Read the model definition and answer for the solid it produces. Units are mm, in the model's axes. Face numbers are marked on the shaded views. A direction names the side the tool comes from. Coordinates: 2 decimals unless noted, no trailing zeros. Loops run counter-clockwise (first coordinate to the right, second up) from the corner with the lowest first, then second, coordinate; pieces in that order, holes last. Notation, with made-up numbers: M 66.5,-20.75 L 71.5,-20.75 A27 ccw 71.5,5.25 Z; hole C -32,29.25 d4. An arc over 180 degrees is marked long. Put each result on its own line as item: value.
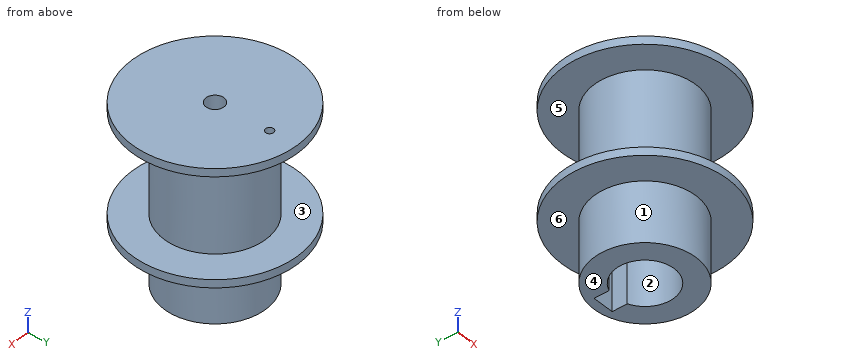
from build123d import *

# Parameters (mm, degrees)
SKETCH1_R           = 12.7
BOSS_EXTRUDE1_DEPTH = 28
SKETCH3_R           = 20.7
SKETCH3_R_2         = 12.7
BOSS_EXTRUDE2_DEPTH = 2
SKETCH4_R           = 12.7
SKETCH4_R_2         = 2.25
BOSS_EXTRUDE3_DEPTH = 14
SKETCH5_R           = 20.7
SKETCH5_R_2         = 2.25
SKETCH5_R_3         = 1
BOSS_EXTRUDE4_DEPTH = 2


with BuildPart() as part:
    # Sketch1 → Boss-Extrude1 (new body)
    with BuildSketch(Plane.XY):
        Circle(SKETCH1_R)
        with BuildLine():
            Line((-2.7, 6.728484228), (-2.7, 10.5))
            Line((-2.7, 10.5), (2.7, 10.5))
            Line((2.7, 10.5), (2.7, 6.728484228))
            ThreePointArc((2.7, 6.728484228), (0, -7.25), (-2.7, 6.728484228))
        make_face(mode=Mode.SUBTRACT)
    extrude(amount=BOSS_EXTRUDE1_DEPTH)

    # Sketch3 → Boss-Extrude2 (add)
    with BuildSketch(Plane(origin=(0, 0, 15), x_dir=(-1, 0, 0), z_dir=(0, 0, -1))):
        Circle(SKETCH3_R)
        Circle(SKETCH3_R_2, mode=Mode.SUBTRACT)
    extrude(amount=-BOSS_EXTRUDE2_DEPTH)

    # Sketch4 → Boss-Extrude3 (add)
    with BuildSketch(Plane.XY.offset(28)):
        with Locations(Location((0, 0, 0), (0, 0, 180))):
            Circle(SKETCH4_R)
        Circle(SKETCH4_R_2, mode=Mode.SUBTRACT)
    extrude(amount=BOSS_EXTRUDE3_DEPTH)

    # Sketch5 → Boss-Extrude4 (add)
    with BuildSketch(Plane.XY.offset(42)):
        with Locations(Location((0, 0, 0), (0, 0, 180))):
            Circle(SKETCH5_R)
        Circle(SKETCH5_R_2, mode=Mode.SUBTRACT)
        with Locations(Location((0, 13.7, 0), (0, 0, 269.999219862))):
            Circle(SKETCH5_R_3, mode=Mode.SUBTRACT)
    extrude(amount=BOSS_EXTRUDE4_DEPTH)


solid = part.part
1) Which of the six approach directions +Z, -Z, +X, -X, +Y, -Y give full straight-line access (tool end or side, diameter ignored) to the marked faces 4, 5 and 6?
Answer list:
face 4: -Z, +X, -X, +Y, -Y
face 5: none
face 6: -Z
2) Given pin 1 Ø6 at (x, z) = (7, 28.5) entering from -Y; pin 2 Ø4 at (y, z) = (-2.5, 31) entering from -X; pin 3 Ø10 at (x, z) = (-5, 21) entering from +Y, each flat-ended and moving along its own axis, determine where each tip first touches the part or whether it passes through.
Answer list:
pin 1: stops at y = -12.05
pin 2: stops at x = -12.69
pin 3: stops at y = 20.6
3) Find section C-C, the plane x = 18.5. Write down the section's boundary in (y, z).
Answer list:
outline: M -9.29,15 L 9.29,15 L 9.29,17 L -9.29,17 Z; M -9.29,42 L 9.29,42 L 9.29,44 L -9.29,44 Z
4) Find section D-D, the plane y = 13.7. Write down the section's boundary in (x, z).
Answer list:
outline: M -15.52,15 L 15.52,15 L 15.52,17 L -15.52,17 Z; M -15.52,42 L -1,42 L -1,44 L -15.52,44 Z; M 1,42 L 15.52,42 L 15.52,44 L 1,44 Z
5) Determine the mould class of the marked faces 1, 2 and 3 for opening direction Y: released by +Y, released by -Y, zero draft, split by the parting line, or undercut.
Answer list:
face 1: split by the parting line
face 2: undercut
face 3: zero draft
6) Find section B-B, the plane z = 3. Write down the section's boundary in (x, y), plus the area to 3 significant figures.
Answer list:
outline: C 0,0 d25.4; hole M -2.7,6.73 A7.25 ccw long 2.7,6.73 L 2.7,10.5 L -2.7,10.5 Z
area: 323 mm^2
7) Straight lines are drawn through the part: line 1 (Z direction, x = 12, y = -16.5); line 2 (X direction, y = 0, z = 23.5); line 3 (X direction, y = 13.7, z = 43.25). For each, find the intervals that lie inside material, in ascending order. Write a range as [from, to].
Answer list:
line 1: z = [15, 17], [42, 44]
line 2: x = [-12.7, -7.25], [7.25, 12.7]
line 3: x = [-15.52, -1], [1, 15.52]
8) Find section A-A, the plane y = -15. Write down the section's boundary in (x, z) (3 decimals), plus the area to 3 significant figures.
Answer list:
outline: M -14.265,15 L 14.265,15 L 14.265,17 L -14.265,17 Z; M -14.265,42 L 14.265,42 L 14.265,44 L -14.265,44 Z
area: 114 mm^2
